The drawing under review shows one solid part. Ordinate dimensions are in mm from its lowest x, y, z. Coordinates: 2 decimals unless noted, no trailing zeros. Write each loop counter-clockwise with the first axis right and the second up, starting at its lowest first coordinate (ties: lowest second). Pieces come first, ordered by that corner, then holes. Notation, with made-up numbers: (-15.5, 20.25) -> (-7.5, 20.25) arc R12 cw to (-7.5, 34.25) -> close; hole circle Ø11 at (31.5, 60). An arc over 180 degrees is marked (long way). One line per question, with ' | ' between items. Start each with the question number.
Q1. Add section B-B on z = 13. State the section outline as (x, y) points.
Q2. Wall thickness on probe 1 along Y at (x, z) = (6.25, 1.5); probe 2 along X at (y, z) = (63, 10.5): over which ranges is each line inside the solid? List them lowest first.
Q3. Add section C-C on y = 62.5. State the section outline as (x, z) points, and give its area (3 significant figures).
Q4. Add section A-A on x = 7. State the section outline as (y, z) points.
Q5. For P1, Ø1, axis at y = 51.5, z = 6, coming from the +X side; P2, Ø6, axis at x = 3.5, y = 51.5, coming from the -Z side; P3, Ø1.5, axis at x = 10, y = 43.5, coming from the -Z side, all flat-tipped, find the tip position at first contact; note any pin that passes through.
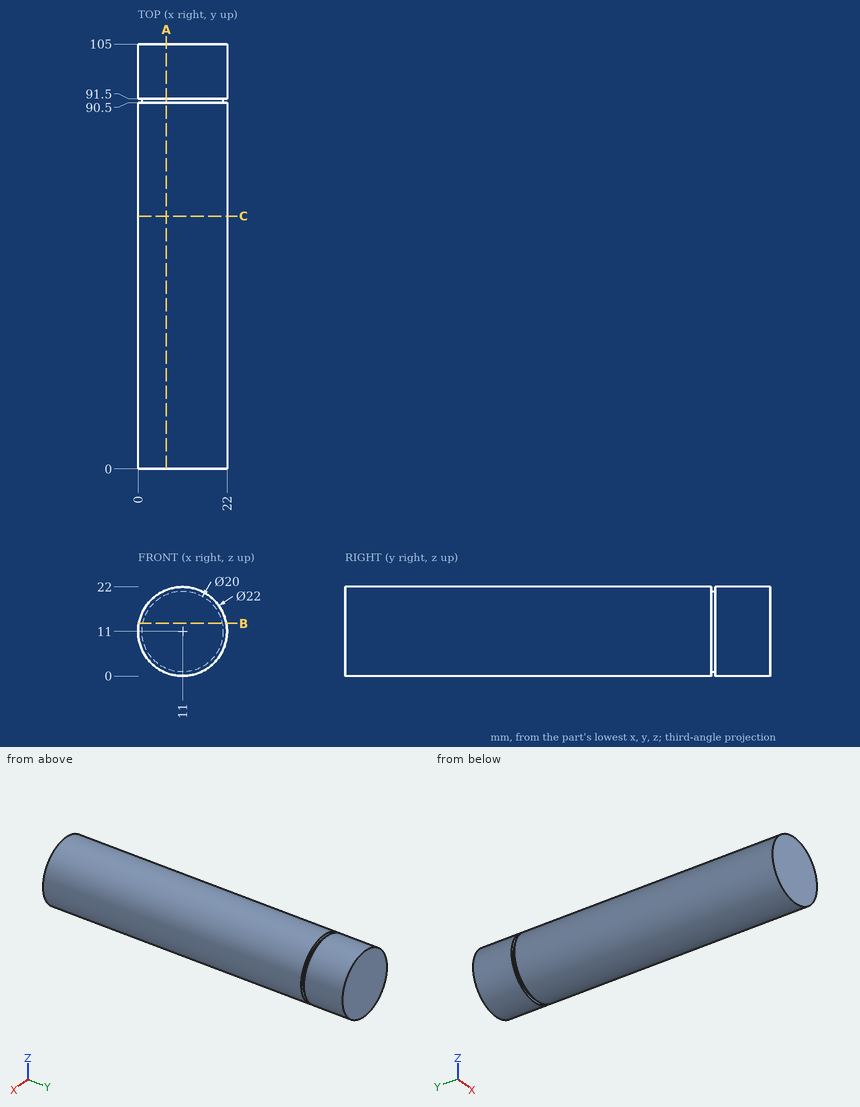
Output values:
1) outline: (0.18, 0) -> (21.82, 0) -> (21.82, 90.5) -> (20.8, 90.5) -> (20.8, 91.5) -> (21.82, 91.5) -> (21.82, 105) -> (0.18, 105) -> (0.18, 91.5) -> (1.2, 91.5) -> (1.2, 90.5) -> (0.18, 90.5) -> close
2) probe 1: y = 0 to 90.5, 91.5 to 105 | probe 2: x = 0.01 to 21.99
3) outline: circle Ø22 at (11, 11) | area: 380 mm2
4) outline: (0, 0.75) -> (90.5, 0.75) -> (90.5, 1.83) -> (91.5, 1.83) -> (91.5, 0.75) -> (105, 0.75) -> (105, 21.25) -> (91.5, 21.25) -> (91.5, 20.17) -> (90.5, 20.17) -> (90.5, 21.25) -> (0, 21.25) -> close
5) P1: stops at x = 21.04 | P2: stops at z = 0.96 | P3: stops at z = 0
